Geometry: final body of the model. Coordinates: model frame, mm. Face numbers are marked on the shaded views. A direction names the side the tool comes from. Round coordinates to 2 decimals unless told otherwise and drop trailing zeros. Loops run counter-clockwise (first coordinate to the right, second up) from the corner with the lowest first, then second, coordinate; pieces in that order, holes last. Notation, with made-up numbers: (-22.5, 13) -> (-13.5, 13) arc R17 cw to (-13.5, 22) -> close; hole circle Ø1 at (47, 34.25). An arc over 180 degrees is marked (long way). Answer in a Markdown table with one row per item.
```python
from build123d import *

# Parameters (mm, degrees)
F0_W     = 19.05
F0_H     = 19.05
F0_W_2   = 15.875
F0_H_2   = 15.875
F1_DEPTH = 57.15
F3_D     = 5.953125
F3_DEPTH = 6.35
F5_D     = 12.7
F5_DEPTH = 6.35
F7_D     = 12.7
F7_DEPTH = 6.35
F9_D     = 5.953125
F9_DEPTH = 6.35


with BuildPart() as f1:
    # F0 (on Front) → F1 (new body)
    with BuildSketch(Plane.XZ):
        Rectangle(F0_W, F0_H)
        Rectangle(F0_W_2, F0_H_2, mode=Mode.SUBTRACT)
    extrude(amount=F1_DEPTH)

    # F3
    with Locations(Plane(origin=(0, 0, -9.525), x_dir=(1, 0, 0), z_dir=(0, 0, -1))):
        with Locations((0, 44.45), (0, 12.7)):
            Hole(F3_D / 2, depth=F3_DEPTH)

    # F5
    with Locations(Plane.XY.offset(9.525)):
        with Locations((0, -12.7), (0, -44.45)):
            Hole(F5_D / 2, depth=F5_DEPTH)

    # F7
    with Locations(Plane.YZ.offset(9.525)):
        with Locations((-28.575, 0)):
            Hole(F7_D / 2, depth=F7_DEPTH)

    # F9
    with Locations(Plane(origin=(-9.525, 0, 0), x_dir=(0, -1, 0), z_dir=(-1, 0, 0))):
        with Locations((28.575, 0)):
            Hole(F9_D / 2, depth=F9_DEPTH)


solid = f1.part
```
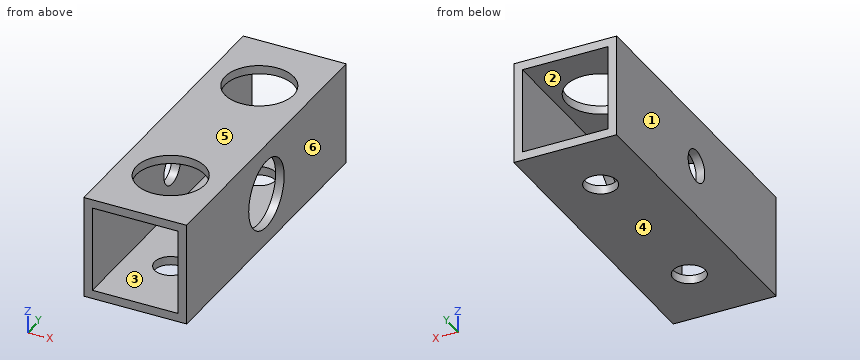
Item 1: First-contact query: P1, Ø5.5, axis at x = 0, y = -12.7, coming from the -Z side; P2, Ø7.5, axis at x = 0, y = -44.45, coming from the +Z side. Flat tips, straight axial feed; report the tip coordinate or a pass-through.
Ans:
| item | result |
|---|---|
| P1 | through |
| P2 | z = -7.94 |
Item 2: Set-up query: the marked faces 1 and 2. Return all of +Z, -Z, +X, -X, +Y, -Y with unobstructed straight access to the full face (end or side cutting, diameter ignored); none if empty.
Ans:
| item | result |
|---|---|
| face 1 | +Z, -Z, -X, +Y, -Y |
| face 2 | +Y, -Y |
Item 3: Section query D-D, the plane y = -24.5. Output: boundary loops of the cut face in (x, z) (1 decimal).
Ans:
| item | result |
|---|---|
| outline | (-9.5, -9.5) -> (9.5, -9.5) -> (9.5, -4.9) -> (7.9, -4.9) -> (7.9, -7.9) -> (-7.9, -7.9) -> (-7.9, 7.9) -> (7.9, 7.9) -> (7.9, 4.9) -> (9.5, 4.9) -> (9.5, 9.5) -> (-9.5, 9.5) -> close |
Item 4: Section query B-B, the plane z = 0. State how many separate pieces and enclosed holes the cut face has, and give its area (3 significant figures).
Ans:
| item | result |
|---|---|
| separate pieces | 4 |
| enclosed holes | 0 |
| area | 152 mm2 |
Item 5: Mould query, pull axis Z, two halves, no side actions, for the marked faces 3, 4, 5 and 6. Classes: released by +Z, released by -Z, zero draft, split by the parting line, or undercut.
Ans:
| item | result |
|---|---|
| face 3 | undercut |
| face 4 | released by -Z |
| face 5 | released by +Z |
| face 6 | zero draft |
Item 6: Ray query, L1, parallel to Y at x = 0, z = -8.7; L2, parallel to Y at x = 0, z = 8.95; L3, parallel to X at y = -31.5, z = -6.5 (1 decimal). Return the intervals inside material, ascending.
Ans:
| item | result |
|---|---|
| L1 | -57.15 to -47.43, -41.47 to -15.68, -9.72 to 0 |
| L2 | -57.15 to -50.8, -38.1 to -19.05, -6.35 to 0 |
| L3 | -9.5 to -7.9, 7.9 to 9.5 |
